```python
from build123d import *

# Parameters (mm, degrees)
SKETCH_1_R      = 29.748261452
EXTRUDE_1_DEPTH = 23
SKETCH_5_W      = 31.165698276
SKETCH_5_H      = 73.42599541
EXTRUDE_4_DEPTH = 90
SKETCH_6_R      = 35.273996594
EXTRUDE_5_DEPTH = 18


with BuildPart() as part:
    # 草图1 → 凸台-拉伸1 (new body)
    with BuildSketch(Plane(origin=(0, 0, 0), x_dir=(1, 0, 0), z_dir=(0, 1, 0))):
        with Locations(Location((0, 0, 0), (0, 0, 270))):
            Circle(SKETCH_1_R)
    extrude(amount=EXTRUDE_1_DEPTH)

    # 草图5 → 凸台-拉伸4 (add)
    with BuildSketch(Plane.XZ):
        Rectangle(SKETCH_5_W, SKETCH_5_H)
    extrude(amount=EXTRUDE_4_DEPTH)

    # 草图6 → 凸台-拉伸5 (add)
    with BuildSketch(Plane(origin=(0, 0, -36.712997705), x_dir=(-1, 0, 0), z_dir=(0, 0, -1))):
        with Locations(Location((0, -43.77696479, 0), (0, 0, 116.216607407))):
            Circle(SKETCH_6_R)
    extrude(amount=EXTRUDE_5_DEPTH)


solid = part.part
```
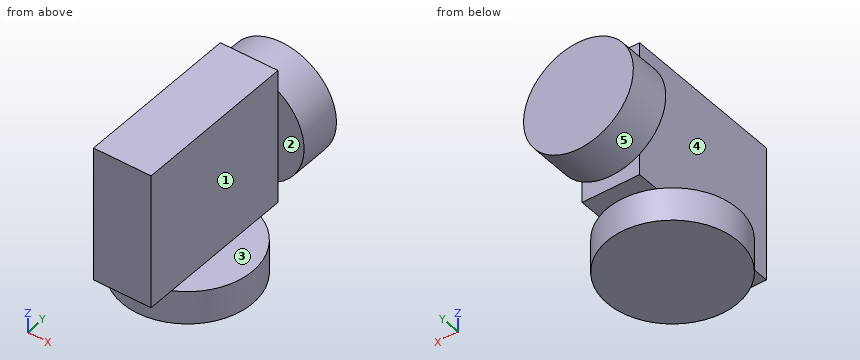
Build history of the part. All positions in model axes, mm. Face numbers are marked on the shaded views. A direction names the side the tool comes from. Give positions to 0.01 mm unless a question says otherwise; leave off trailing zeros. Loops run counter-clockwise (first coordinate to the right, second up) from the corner with the lowest first, then second, coordinate; pieces in that order, holes last. Notation, with made-up numbers: (-29, 48.25) -> (-9, 48.25) arc R15 ccw to (-9, 55.25) -> close; hole circle Ø2 at (88.5, -9.75). An arc over 180 degrees is marked (long way). One line per question, with ' | ' between items. Start each with the question number.
1) Cut at A-A (x = 21). Give the cut face in (y, z).
2) 3-axis set-ups, long thin cutter, end or side, ignore diameter. For the marked faces 1, 2, 3, 4 and 5: which of +Z, -Z, +X, -X, +Y, -Y reach the whole face in a straight line?
3) Cut at D-D (x = 0). Give the cut face in (y, z).
4) Cut at C-C (y = -13.5). Give the cut face in (x, z).
5) Pin check, flat tips, straight feed: pin 1 (3 mm diameter, centred on y = 2.5, z = 11.5, fed in from -X); pin 2 (3.5 mm diameter, centred on x = -5, z = 32.5, fed in from +Y); pin 3 (8 mm diameter, centred on x = 27.5, z = -31, fed in from -Y); pin 4 (11.5 mm diameter, centred on x = 3, y = -86, fed in from -Z). Stop position of each tip, or through.
6) Cut at B-B (z = 0). Give the cut face in (x, y).
7) Probe L1, parallel to X at y = -6, z = 31.5; L2, parallel to Z at x = 25, y = -59.5; L3, parallel to Y at x = 1, z = -38. List the from-to ranges inside material, lowest first.
Return value:
1) outline: (-72.12, -54.71) -> (-15.44, -54.71) -> (-15.44, -36.71) -> (-72.12, -36.71) -> close; (0, -21.07) -> (23, -21.07) -> (23, 21.07) -> (0, 21.07) -> close
2) face 1: +Z, +X, -Y | face 2: +Z, -Z, +X, -Y | face 3: +Z, +X, +Y, -Y | face 4: +Z, -X, -Y | face 5: +Y
3) outline: (-90, -36.71) -> (-79.05, -36.71) -> (-79.05, -54.71) -> (-8.5, -54.71) -> (-8.5, -36.71) -> (0, -36.71) -> (0, -29.75) -> (23, -29.75) -> (23, 29.75) -> (0, 29.75) -> (0, 36.71) -> (-90, 36.71) -> close
4) outline: (-18.1, -54.71) -> (18.1, -54.71) -> (18.1, -36.71) -> (15.58, -36.71) -> (15.58, 36.71) -> (-15.58, 36.71) -> (-15.58, -36.71) -> (-18.1, -36.71) -> close
5) pin 1: x = -28.02 | pin 2: y = 0 | pin 3: through | pin 4: z = -36.71
6) outline: (-29.75, 0) -> (-15.58, 0) -> (-15.58, -90) -> (15.58, -90) -> (15.58, 0) -> (29.75, 0) -> (29.75, 23) -> (-29.75, 23) -> close
7) L1: -15.58 to 15.58 | L2: -54.71 to -36.71 | L3: -79.04 to -8.52
